Check sheet for the modelled part. Datum: model origin and axes. Units: mm. A direction names the side the tool comes from. Round coordinates to 2 decimals unless told otherwise and drop trailing zeros. Loops run counter-clockwise (first coordinate to the right, second up) from the corner with the lowest first, then second, coordinate; pieces in that order, holes last. Notation, with made-up numbers: (7.5, -9.5) -> (27.5, -9.5) arc R21 ccw to (27.5, 17.5) -> close; hole circle Ø3 at (78, -17). An arc over 180 degrees is marked (long way). One line per item, written item: value. Start each with the question number.
1. Cross-section at A-A on x = 0. Record the cut outline in (y, z) (1 decimal).
2. Set-up check for faces 1 (the face through (8, 3, 1.27)), 2 (the face through (0, 2, -4.762)), 3 (the face through (-8, 3, -1.27)): record each of +Z, -Z, +X, -X, +Y, -Y from which the full face is reachable in a straight line by a thin tool's end or side.
3. Cross-section at C-C on z = 0. Record the cut outline in (x, y) (1 decimal), then the cut area to 3 significant figures.
4. Material ranges on L1, parallel to Z at x = 5, y = 2.85; L2, parallel to Z at x = 0, y = 2.2; L3, parallel to Y at x = -7.5, z = 0 (3 decimals), recorded low to high.
5. Go/stop test with a flat-tipped pin: pin 1 (1.4 mm diameter, centred on x = 0, z = 0, fed in from -Y). Record where the tip stops, or that it passes through.
6. Cross-section at B-B on y = 2.35. Record the cut outline in (x, z).
7. Release check for a two-part mould opening along Z. For faces 4 (the face through (0, 2, 4.762)), 5 (the face through (8, 1.905, 0)), 6 (the face through (14.288, 1.6, 0.1)) record: +Z half, -Z half, draft (parallel to the pull), parting line (faces both ways), or undercut.
8. Cross-section at D-D on x = 10. Record the cut outline in (y, z) (1 decimal), then the cut area to 3 significant figures.
from build123d import *

# Parameters (mm, degrees)
SKETCH1_W                 = 28.575
SKETCH1_H                 = 9.525
BOSS_EXTRUDE1_DEPTH       = 3.175
F_4_40_TAPPED_HOLE1_D     = 2.2606
F_4_40_TAPPED_HOLE1_DEPTH = 7.5946
F_4_40_TAPPED_HOLE1_TIP   = 0.679152758
SKETCH5_W                 = 12.5095
SKETCH5_H                 = 2.54
CUT_EXTRUDE2_DEPTH        = 1.27


with BuildPart() as part:
    # Sketch1 → Boss-Extrude1 (new body)
    with BuildSketch(Plane(origin=(0, 0, 0), x_dir=(1, 0, 0), z_dir=(0, 1, 0))):
        Rectangle(SKETCH1_W, SKETCH1_H)
    extrude(amount=BOSS_EXTRUDE1_DEPTH)

    # #4-40 Tapped Hole1
    with Locations(Plane(origin=(0, 3.175, 0), x_dir=(1, 0, 0), z_dir=(0, 1, 0))):
        with Locations((0, 0)):
            Hole(F_4_40_TAPPED_HOLE1_D / 2, depth=F_4_40_TAPPED_HOLE1_DEPTH)
            with Locations((0, 0, -(F_4_40_TAPPED_HOLE1_DEPTH + F_4_40_TAPPED_HOLE1_TIP / 2))):  # 118° drill point
                Cone(0, F_4_40_TAPPED_HOLE1_D / 2, F_4_40_TAPPED_HOLE1_TIP, mode=Mode.SUBTRACT)

    # Sketch5 → Cut-Extrude2 (cut)
    with BuildSketch(Plane(origin=(0, 3.175, 0), x_dir=(1, 0, 0), z_dir=(0, 1, 0))):
        with Locations((-8.03275, 0)):
            Rectangle(SKETCH5_W, SKETCH5_H)
        with Locations((8.03275, 0)):
            Rectangle(SKETCH5_W, SKETCH5_H)
    extrude(amount=-CUT_EXTRUDE2_DEPTH, mode=Mode.SUBTRACT)


solid = part.part
Taken from the geometry:
1. outline: (0, -4.8) -> (3.2, -4.8) -> (3.2, -1.1) -> (0, -1.1) -> close; (0, 1.1) -> (3.2, 1.1) -> (3.2, 4.8) -> (0, 4.8) -> close
2. face 1: +X, +Y
2. face 2: -Z, +X, -X, +Y, -Y
2. face 3: -X, +Y
3. outline: (-14.3, 0) -> (-1.1, 0) -> (-1.1, 3.2) -> (-1.8, 3.2) -> (-1.8, 1.9) -> (-14.3, 1.9) -> close; (1.1, 0) -> (14.3, 0) -> (14.3, 1.9) -> (1.8, 1.9) -> (1.8, 3.2) -> (1.1, 3.2) -> close
3. area: 51.8 mm2
4. L1: z = -4.76 to -1.27, 1.27 to 4.76
4. L2: z = -4.76 to -1.13, 1.13 to 4.76
4. L3: y = 0 to 1.905
5. pin 1: passes through
6. outline: (-14.29, -4.76) -> (14.29, -4.76) -> (14.29, -1.27) -> (1.78, -1.27) -> (1.78, 1.27) -> (14.29, 1.27) -> (14.29, 4.76) -> (-14.29, 4.76) -> (-14.29, 1.27) -> (-1.78, 1.27) -> (-1.78, -1.27) -> (-14.29, -1.27) -> close; hole circle Ø2.26 at (0, 0)
7. face 4: +Z half
7. face 5: undercut
7. face 6: draft
8. outline: (0, -4.8) -> (3.2, -4.8) -> (3.2, -1.3) -> (1.9, -1.3) -> (1.9, 1.3) -> (3.2, 1.3) -> (3.2, 4.8) -> (0, 4.8) -> close
8. area: 27.0 mm2
